```python
from build123d import *

# Parameters (mm, degrees)
F1_DEPTH      = 11
F1_DEPTH_BACK = 11
F2_R          = 10
F3_DEPTH      = 25
F6_END_RADIUS = 13.15
F5_R          = 12
F5_R_2        = 10
F6_REACH      = 68.442125597
F7_T4_ANGLE   = 86.3533795546
F7_S5_R       = 12
F7_T6_DEPTH   = 12
F8_W          = 15.702219009
F8_H          = 5.1735627732
F9_DEPTH      = 32.5010001


# Not quite as in the source:
# - a fillet or chamfer that OpenCascade refuses, or shapes differently, is made with other operations: its cross-section is extruded or revolved along the edge and cut away or added


with BuildPart() as f1:
    # F0 (on Top) → F1 (new body, two sides)
    with BuildSketch(Plane.XY) as f1_sk:
        with BuildLine():
            ThreePointArc((-1.4356223176, 11.0571917122), (11.15, 0), (-1.4356223176, -11.0571917122))
            ThreePointArc((-1.4356223176, -11.0571917122), (-1.8300084535, -11.1774045329), (-2, -11.5530299056))
            Line((-2, -11.5530299056), (-2, -12.997018889))
            ThreePointArc((-2, -12.997018889), (13.15, 0), (-2, 12.997018889))
            Line((-2, 12.997018889), (-2, 11.5530299056))
            ThreePointArc((-2, 11.5530299056), (-1.8300084535, 11.1774045329), (-1.4356223176, 11.0571917122))
        make_face()
    extrude(amount=F1_DEPTH)
    extrude(f1_sk.sketch, amount=-F1_DEPTH_BACK)

    # F2 (on Right) → F3 (cut)
    with BuildSketch(Plane.YZ):
        Circle(F2_R)
    extrude(amount=F3_DEPTH, mode=Mode.SUBTRACT)

    f6_end = (Plane(origin=(0, 0, 0), x_dir=(-1, 0, 0), z_dir=(0, 0, -1)) * Cylinder(F6_END_RADIUS, 211.856580101, mode=Mode.PRIVATE)).faces().sort_by_distance((13.15, 0, 10.6251383555))[0]
    # F5 (on offset) → F6 (join, up to the whole of a round face its end follows)
    with BuildSketch(Plane.YZ.offset(32.5)):
        Circle(F5_R)
        Circle(F5_R_2, mode=Mode.SUBTRACT)
    f6_long = extrude(amount=-F6_REACH, mode=Mode.PRIVATE)
    add(split(f6_long, bisect_by=f6_end, keep=Keep.ALL, mode=Mode.PRIVATE).solids().sort_by_distance((32.5, -11.660588745, 0))[0])

    # F7: fillet of radius 2 on 1 edges, made by hand


with BuildPart() as f7_tool2:
    # F7_s3 → F7_t4 (revolve)
    with BuildSketch(Plane(origin=(0, 0, 0), x_dir=(0, 0, 1), z_dir=(-0.6842504755, -0.7292470684, 0))):
        with BuildLine():
            ThreePointArc((-11, -11.15), (-11.5857864376, -12.5642135624), (-13, -13.15))
            Line((-13, -13.15), (-11, -13.15))
            Line((-11, -13.15), (-11, -11.15))
        make_face()
    revolve(axis=Axis((0, 0, -11), (0, 0, 1)), revolution_arc=F7_T4_ANGLE)

    # F7_s5 → F7_t6 (intersect, symmetric)
    with BuildSketch(Plane.YZ.offset(10.7)):
        Circle(F7_S5_R)
    extrude(amount=F7_T6_DEPTH, both=True, mode=Mode.INTERSECT)


with BuildPart() as f1_1:
    add(f1.part)

    # F7_t1: union F7_tool2
    add(f7_tool2.part)

    # F8 (on Right) → F9 (cut, through all)
    with BuildSketch(Plane.YZ):
        with Locations((0.481082825, 13.5867813866)):
            Rectangle(F8_W, F8_H)
    extrude(amount=F9_DEPTH, mode=Mode.SUBTRACT)


solid = f1_1.part
```
Part model, mm, in its own coordinate system. A direction names the side the tool comes from. Give positions to 0.01 mm unless a question says otherwise; leave off trailing zeros. Order: outer loops, then holes, each group sorted by start corner. A loop starts at its lowest first (then second) coordinate and runs counter-clockwise, first axis right, second up. Notation, with made-up numbers: (79.25, 58) - (129.25, 58) arc R35 cw to (129.25, 92) - close; hole circle Ø8 at (-22, -10.75). An arc over 180 degrees is marked (long way). Use one line per item in the form item = value.
Item 1: Slice it at C-C on z = -2. Give the cut face in (x, y), and give its area (3 significant figures).
Solution:
outline = (-2, -13) arc R13.15 ccw to (5.74, -11.83) - (32.5, -11.83) - (32.5, -9.8) - (5.32, -9.8) arc R11.15 cw to (-1.44, -11.06) arc R0.5 ccw to (-2, -11.55) - close; (-2, 11.55) arc R0.5 ccw to (-1.44, 11.06) arc R11.15 cw to (5.32, 9.8) - (32.5, 9.8) - (32.5, 11.83) - (5.74, 11.83) arc R13.15 ccw to (-2, 13) - close
area = 141 mm2
Item 2: Two-plate mould, pull along Y, no slides. Class faces 1 (the face through (3.02, 12.8, 0.15)), 2 (the face through (6, 10, -11)), 3 (the face through (4.5, 10.2, 0.2)): released by +Y, released by -Y, zero draft, split by the parting line, or undercut.
Solution:
face_1 = released by +Y
face_2 = zero draft
face_3 = undercut
Item 3: Pin check, flat tips, straight feed: pin 1 Ø3 at (x, z) = (18.5, -4.5) entering from -Y; pin 2 Ø10 at (x, z) = (27.5, 5) entering from -Y; pin 3 Ø2.5 at (x, y) = (5.5, 11) entering from -Z; pin 4 Ø4 at (y, z) = (-5, -8) entering from +X. Stop position of each tip, or through.
Solution:
pin_1 = -11.62
pin_2 = -12
pin_3 = -11
pin_4 = 32.5
Item 4: Slice it at B-B on x = 0. Give the cut face in (y, z), and give its area (3 significant figures).
Solution:
outline = (-13.15, -11) - (-11.15, -11) - (-11.15, 11) - (-13.15, 11) - close; (11.15, -11) - (13.15, -11) - (13.15, 11) - (11.15, 11) - close
area = 88.0 mm2
Item 5: Which spindle directions (+Z, -Z, +X, -X, +Y, -Y) get a long thin tool onto all of the face, cutting with end or side? Do faces 4 (the face through (6, -10, -11)), 5 (the face through (2.779, -12.853, 0.154)), 6 (the face through (18, -1, 11)). Say none if no direction does.
Solution:
face_4 = -Z, +X, -X, -Y
face_5 = -Y
face_6 = +Z, +X, -X, +Y, -Y
Item 6: Probe probe 1 along Y at (x, z) = (14, 0); probe 2 along Z at (x, y) = (20.5, 0); probe 3 along Y at (x, z) = (6, -8). List the from-to ranges inside material, lowest first. Write a range as from..to.
Solution:
probe_1 = -12..-10, 10..12
probe_2 = -12..-10, 10..11
probe_3 = -11.7..-9.4, 9.4..11.7
Item 7: Slice it at D-D on x = 20. Give the cut face in (y, z), and give its area (3 significant figures).
Solution:
outline = (-4.8, 11) arc R12 ccw (long way) to (4.8, 11) - close; hole circle Ø20 at (0, 0)
area = 132 mm2
Item 8: Slice it at A-A on y = 0. Give the cut face in (x, z), and give its area (3 significant figures).
Solution:
outline = (11.15, -11) arc R2 cw to (12.88, -12) - (32.5, -12) - (32.5, -10) - (11.15, -10) - close; (11.15, 10) - (32.5, 10) - (32.5, 11) - (11.15, 11) - close
area = 62.8 mm2
